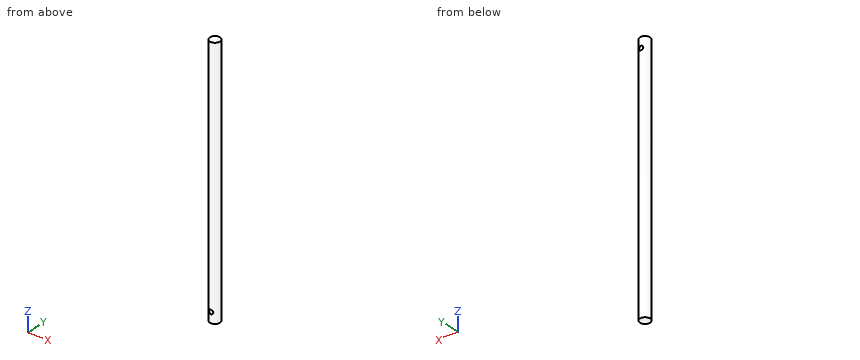
```python
from build123d import *

# Parameters (mm, degrees)
ESQUISSE1_R             = 0.5
BOSS_EXTRU_1_DEPTH      = 25
ESQUISSE3_R             = 0.2
ENL_V_MAT_EXTRU_3_DEPTH = 1
ESQUISSE4_R             = 0.2
ENL_V_MAT_EXTRU_4_DEPTH = 1


with BuildPart() as part:
    # Esquisse1 → Boss.-Extru.1 (new body)
    with BuildSketch(Plane.XY):
        Circle(ESQUISSE1_R)
    extrude(amount=BOSS_EXTRU_1_DEPTH)

    # Esquisse3 → Enlèv. mat.-Extru.3 (cut)
    with BuildSketch(Plane(origin=(0, 0, 0), x_dir=(1, 0, 0), z_dir=(0, 1, 0))):
        with Locations((0, -1)):
            Circle(ESQUISSE3_R)
    extrude(amount=-ENL_V_MAT_EXTRU_3_DEPTH, mode=Mode.SUBTRACT)

    # Esquisse4 → Enlèv. mat.-Extru.4 (cut)
    with BuildSketch(Plane(origin=(0, 0, 0), x_dir=(1, 0, 0), z_dir=(0, 1, 0))):
        with Locations((0, -24)):
            Circle(ESQUISSE4_R)
    extrude(amount=ENL_V_MAT_EXTRU_4_DEPTH, mode=Mode.SUBTRACT)


solid = part.part
```
Geometry check sheet. Reference: the model listing, model coordinates, mm. Give positions to 0.01 mm unless a question says otherwise; leave off trailing zeros. Write each loop counter-clockwise with the first axis right and the second up, starting at its lowest first coordinate (ties: lowest second). Pieces come first, ordered by that corner, then holes. Notation, with made-up numbers: (-36, -40) - (-13, -40) arc R30 cw to (-13, -10) - close; hole circle Ø9 at (-8.5, 67.25). An arc over 180 degrees is marked (long way). Use a Markdown table: item, result.
Q1. Section check A-A, the plane x = 0. Enter the section's corners in (y, z), then the cut area to 3 significant figures.
Computed:
| item | result |
|---|---|
| outline | (-0.5, 0) - (0.5, 0) - (0.5, 23.8) - (0, 23.8) - (0, 24.2) - (0.5, 24.2) - (0.5, 25) - (-0.5, 25) - (-0.5, 1.2) - (0, 1.2) - (0, 0.8) - (-0.5, 0.8) - close |
| area | 24.6 mm² |
Q2. Thickness scan on L1, parallel to Z at x = 0, y = 0.05; L2, parallel to Z at x = 0, y = -0.25; L3, parallel to X at y = -0.25, z = 1. Record the ranges inside material, lowest first. Write a range as [from, to].
Computed:
| item | result |
|---|---|
| L1 | z = [0, 23.8], [24.2, 25] |
| L2 | z = [0, 0.8], [1.2, 25] |
| L3 | x = [-0.43, -0.2], [0.2, 0.43] |
Q3. Section check B-B, the plane y = -0.2. Enter the section's corners in (x, z).
Computed:
| item | result |
|---|---|
| outline | (-0.46, 0) - (0.46, 0) - (0.46, 25) - (-0.46, 25) - close; hole circle Ø0.4 at (0, 1) |
Q4. Section check C-C, the plane z = 10.75. Enter the section's corners in (x, y), then the cut area to 3 significant figures.
Computed:
| item | result |
|---|---|
| outline | circle Ø1 at (0, 0) |
| area | 0.785 mm² |
